Autodesk Inventor part; units mm, degrees
ref_plane "YZ Plane" through (0, 0, 0) normal (1, 0, 0) x (0, 1, 0)
ref_plane "XZ Plane" through (0, 0, 0) normal (0, 1, 0) x (-1, 0, 0)
ref_plane "XY Plane" through (0, 0, 0) normal (0, 0, 1) x (1, 0, 0)
sketch "Sketch1" plane through (0, 0, 0) normal (0, 0, 1) x (1, 0, 0)
  circle A0 centre (0, 0) radius 4
  circle A1 centre (0, 0) radius 2
  line L0 (0, -4) -> (6, -4)
  line L1 (6, -4) -> (6, 4)
  line L2 (6, 4) -> (0, 4)
  circle A2 centre (22, 0) radius 2.5
  circle A3 centre (22, 0) radius 3
  line L3 (22, -3) -> (16, -3)
  line L4 (16, -3) -> (16, 3)
  line L5 (16, 3) -> (22, 3)
  line L6 (16, -2) -> (6, -2)
  line L7 (6, 2) -> (16, 2)
  dimension "d0" = 8
  dimension "d1" = 4
  dimension "d8" = 6
  dimension "d9" = 5
  dimension "d10" = 6
  dimension "d11" = 6
  dimension "d12" = 6
  dimension "d17" = 10
  dimension "d19" = 4
extrude "Extrusion1" add sketch "Sketch1" along normal blind 3
fillet "Fillet1" radius 8 1 edges at (6, -2, 1.5)
fillet "Fillet2" radius 8 3 edges at (6, 2, 1.5) (16, 2, 1.5) (16, -2, 1.5)
properties part number "PLEUEL short new"
Part model, mm, in its own coordinate system. A direction names the side the tool comes from. Give positions to 0.01 mm unless a question says otherwise; leave off trailing zeros. Order: outer loops, then holes, each group sorted by start corner. A loop starts at its lowest first (then second) coordinate and runs counter-clockwise, first axis right, second up. Notation, with made-up numbers: (-8, 13.25) -> (43, 13.25) arc R24 cw to (43, 38.25) -> close; hole circle Ø5 at (49, -7.5). An arc over 180 degrees is marked (long way). Use one line per item in the form item = value.
(1) Pull direction X, two halves, no side cores. Call faces 4 (the face through (25, 0, 1)), 5 (the face through (-4, 0, 1)), 6 (the face through (11.7, -2, 1.5)): +X half, -X half, draft (parallel to the pull), parting line (faces both ways), or undercut.
Solution:
face_4 = +X half
face_5 = -X half
face_6 = undercut
(2) Drill centre lines: line 1 (Y direction, x = 22, z = 1.1); line 2 (X direction, y = -1.25, z = 2.15); line 3 (X direction, y = 0.75, z = 0.55). Where is each one in solid material? Low to high. Write a range as from..to.
Solution:
line_1 = -3..-2.5, 2.5..3
line_2 = -3.8..-1.56, 1.56..19.83, 24.17..24.73
line_3 = -3.93..-1.85, 1.85..19.62, 24.38..24.9
(3) Saw through at C-C (z = 2.7). Write the cut outline in (x, y), then the cut area to 3 significant figures.
Solution:
outline = (0, -4) -> (6, -4) arc R8 cw to (11.29, -2) -> (12.13, -2) arc R8 cw to (16, -3) -> (22, -3) arc R3 ccw to (22, 3) -> (16, 3) arc R8 cw to (12.13, 2) -> (11.29, 2) arc R8 cw to (6, 4) -> (0, 4) arc R4 ccw to start; hole circle Ø4 at (0, 0); hole circle Ø5 at (22, 0)
area = 140 mm²
(4) Tool access for faces 1 (the face through (19, -3, 1)), 2 (the face through (19, 3, 1)), 3 (the face through (14.15, 2.26, 1.48)): list every direction of +Z, -Z, +X, -X, +Y, -Y with a clear straight run to the whole face (end or side of a thin tool).
Solution:
face_1 = +Z, -Z, +X, -Y
face_2 = +Z, -Z, +X, +Y
face_3 = +Z, -Z, +Y
(5) Saw through at D-D (y = -1.75). Write the cut outline in (x, z).
Solution:
outline = (-3.6, 0) -> (-0.97, 0) -> (-0.97, 3) -> (-3.6, 3) -> close; (0.97, 0) -> (20.21, 0) -> (20.21, 3) -> (0.97, 3) -> close; (23.79, 0) -> (24.44, 0) -> (24.44, 3) -> (23.79, 3) -> close
(6) Flat gauge pins, fed straight in: P1, Ø0.9, axis at x = 20.5, z = 2, coming from the +Y side; P2, Ø3.5, axis at x = 0, y = 0, coming from the +Z side; P3, Ø0.9, axis at x = 12, z = 1.5, coming from the +Y side. Where does each tip first touch, or does it go through?
Solution:
P1 = 3
P2 = through
P3 = 2.01
(7) Saw through at A-A (y = 0). Write the cut outline in (x, z).
Solution:
outline = (-4, 0) -> (-2, 0) -> (-2, 3) -> (-4, 3) -> close; (2, 0) -> (19.5, 0) -> (19.5, 3) -> (2, 3) -> close; (24.5, 0) -> (25, 0) -> (25, 3) -> (24.5, 3) -> close
(8) Saw through at B-B (x = 1.5). Write the cut outline in (y, z), then the cut area to 3 significant figures.
Solution:
outline = (-4, 0) -> (-1.32, 0) -> (-1.32, 3) -> (-4, 3) -> close; (1.32, 0) -> (4, 0) -> (4, 3) -> (1.32, 3) -> close
area = 16.1 mm²
